Design review of the part shown in the three views and the two pictorial views. Dimensions are in mm from the part's minimum x, y and z. Coordinates: 2 decimals unless noted, no trailing zeros. Loops run counter-clockwise (first coordinate to the right, second up) from the corner with the lowest first, then second, coordinate; pieces in that order, holes last.
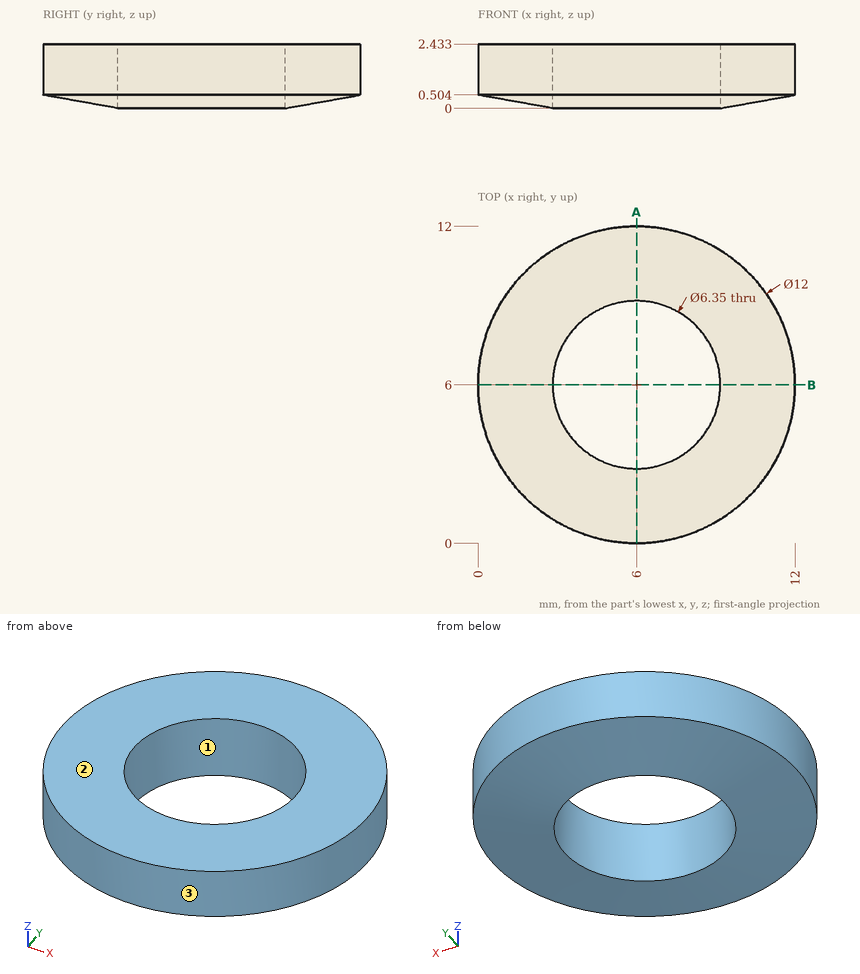
Q1. The part is to be moulded in two halves that separate along X. For the marked faces 1, 2 and 3, say which applies: +X half, -X half, draft (parallel to the pull), parting line (faces both ways), or undercut.
Q2. Consider section A-A (x = 6). State the section outline as (y, z) points (1 decimal).
Q3. Wall thickness on probe 1 along Y at (x, z) = (6, 1.65) (1 decimal); probe 2 along X at (y, z) = (8, 1.35) (1 decimal); probe 3 along Y at (x, z) = (5.5, 1) (1 decimal): over which ranges is each line inside the solid? List them lowest first.
Model answer:
1. face 1: undercut
1. face 2: draft
1. face 3: parting line
2. outline: (0, 0.5) - (2.8, 0) - (2.8, 2.4) - (0, 2.4) - close; (9.2, 0) - (12, 0.5) - (12, 2.4) - (9.2, 2.4) - close
3. probe 1: y = 0 to 2.8, 9.2 to 12
3. probe 2: x = 0.3 to 3.5, 8.5 to 11.7
3. probe 3: y = 0 to 2.9, 9.1 to 12
